Part model, mm, in its own coordinate system. A direction names the side the tool comes from. Round coordinates to 2 decimals unless told otherwise and drop trailing zeros. Loops run counter-clockwise (first coordinate to the right, second up) from the corner with the lowest first, then second, coordinate; pieces in that order, holes last.
from build123d import *

# Parameters (mm, degrees)
BOSS_EXTRUDE1_DEPTH = 12.7


with BuildPart() as part:
    # Sketch1 → Boss-Extrude1 (new body)
    with BuildSketch(Plane(origin=(0, 0, 0), x_dir=(0, 0, -1), z_dir=(1, 0, 0))):
        Polygon((-394.946506416, 268.859), (-444.5, 0), (-424.843977237, 0), (-388.508616862, 197.142278951), (-266.964417858, 95.154586396), (-186.461552382, 27.604661666), (-98.092418556, 0), (-75.979077973, 0), (-73.675108156, -0.719711788), align=None)
        with BuildLine():
            Line((-375.052513862, 235.58728561), (-170.667115901, 64.087573564))
            ThreePointArc((-170.667115901, 64.087573564), (-169.101754117, 46.195406493), (-186.993921187, 44.630044709))
            Line((-186.993921187, 44.630044709), (-391.379319148, 216.129756755))
            ThreePointArc((-391.379319148, 216.129756755), (-392.944680933, 234.021923826), (-375.052513862, 235.58728561))
        make_face(mode=Mode.SUBTRACT)
    extrude(amount=BOSS_EXTRUDE1_DEPTH)


solid = part.part
1) Wall check: line 1 along Z through (x, y) = (8, 176); line 2 along Z through (x, y) = (5.5, 106); line 3 along Y through (x, z) = (2.75, 189). Give the ranges that are in metal, low to high.
Values:
line 1: z = 284.28 to 304.04, 343.55 to 363.31, 392.41 to 412.06
line 2: z = 200.86 to 220.62, 260.13 to 279.89, 405.31 to 424.96
line 3: y = 29.73 to 46.31, 79.47 to 96.05
2) Slice it at C-C, the plane x = 2.75. Give the cut face in (y, z).
Values:
outline: (-0.72, 73.68) - (268.86, 394.95) - (0, 444.5) - (0, 424.84) - (197.14, 388.51) - (27.6, 186.46) - (0, 98.09) - (0, 75.98) - close; hole (44.63, 186.99) arc R12.7 ccw to (64.09, 170.67) - (235.59, 375.05) arc R12.7 ccw to (216.13, 391.38) - close
3) Slice it at A-A, the plane y = 20. Give the cut face in (x, z).
Values:
outline: (0, 98.37) - (12.7, 98.37) - (12.7, 162.12) - (0, 162.12) - close; (0, 421.16) - (12.7, 421.16) - (12.7, 440.81) - (0, 440.81) - close
4) Drop flat-ended pins along their axis: pin 1 Ø4 at (x, z) = (6, 439) entering from -Y; pin 2 Ø1.5 at (x, z) = (8, 125) entering from -Y; pin 3 Ø1 at (x, z) = (3.5, 371) entering from +Y. Give the stop position or say it passes through.
Values:
pin 1: stops at y = 0
pin 2: stops at y = 8.17
pin 3: stops at y = 249.19
5) Mould opens along Z. For faces 1 (the face through (6, 0, 435)), 2 (the face through (6.26, 233.81, 393.12)), 3 (the face through (6.26, 132.18, 232.06)) say: released by +Z, released by -Z, zero draft, split by the parting line, or undercut.
Values:
face 1: zero draft
face 2: undercut
face 3: released by -Z
6) Slice it at B-B, the plane z = 202.5. Give the cut face in (x, y).
Values:
outline: (0, 41.06) - (12.7, 41.06) - (12.7, 57.64) - (0, 57.64) - close; (0, 90.8) - (12.7, 90.8) - (12.7, 107.38) - (0, 107.38) - close
7) Tool access for faces 4 (the face through (6.26, 97.19, 406.93)), 5 (the face through (6.26, 151.04, 274.29)), 6 (the face through (6, 0, 87)): list every direction of +Z, -Z, +X, -X, +Y, -Y with a clear straight run to the whole face (end or side of a thin tool).
Values:
face 4: +X, -X, -Y
face 5: +X, -X
face 6: +Z, +X, -X, -Y
8) Slice it at D-D, the plane y = 51. Give the cut face in (x, z).
Values:
outline: (0, 135.31) - (12.7, 135.31) - (12.7, 166.58) - (0, 166.58) - close; (0, 194.59) - (12.7, 194.59) - (12.7, 214.34) - (0, 214.34) - close; (0, 415.44) - (12.7, 415.44) - (12.7, 435.1) - (0, 435.1) - close
